For this review, take the finished solid that the model builds, in its own axes (mm). Round coordinates to 2 decimals unless told otherwise and drop trailing zeros. Order: outer loops, then holes, each group sorted by start corner. A loop starts at its lowest first (then second) coordinate and runs counter-clockwise, first axis right, second up. Notation, with made-up numbers: (79.25, 76.25) -> (133.25, 76.25) arc R32 ccw to (133.25, 113.25) -> close; hole circle Ø3 at (46, 35). An arc over 180 degrees is marked (long way). Use a Markdown table: item, result. Add a question column.
1) Consider section C-C (x = -23). State the section outline as (y, z) points.
2) Wall thickness on line 1 along Y through (x, z) = (-12.5, 5); line 2 along X through (y, z) = (-17, 3.45); line 3 along Y through (x, z) = (-3, 2.75): over which ranges is each line inside the solid? List them lowest first. Write a range as [from, to].
3) Consider section B-B (y = -16). State the section outline as (x, z) points, plus the area to 3 significant figures.
4) Consider section A-A (z = 3.65). State the section outline as (x, y) points, plus the area to 3 significant figures.
5) Clearance check with flat-ended pins moving along their axes: P1, Ø2, axis at y = 22, z = 2, coming from the +X side; P2, Ø12, axis at x = 21.65, y = -12.5, coming from the +Z side. State where each tip first meets the part, or that it passes through.
6) Draft analysis for pull direction X (two halves, no side actions). For faces 1 (the face through (-29.55, -18.55, 2.96)), 2 (the face through (3, 11, 6)), 3 (the face through (13.75, -18.55, 2.96)), state which applies: pulls with the +X half, pulls with the -X half, needs draft (parallel to the pull), parting line crosses it, or undercut.
7) Consider section D-D (y = 7). State the section outline as (x, z) points, plus the area to 3 significant figures.
```python
from build123d import *

# Parameters (mm, degrees)
F0_R     = 9.95
F1_DEPTH = 6


with BuildPart() as f1:
    # F0 (on Top) → F1 (new body)
    with BuildSketch(Plane.XY):
        with BuildLine():
            ThreePointArc((0, 11), (-7.778175, -7.778175), (11, 0))
            ThreePointArc((11, 0), (7.778175, 7.778175), (0, 11))
        make_face()
        with BuildLine():
            ThreePointArc((9.95, 25), (-7.035712, 32.035712), (0, 15.05))
            ThreePointArc((0, 15.05), (7.035712, 17.964288), (9.95, 25))
        make_face()
        with BuildLine():
            ThreePointArc((8.291562, 12.5), (0, 40), (-8.291562, 12.5))
            ThreePointArc((-8.291562, 12.5), (-12.990381, 7.5), (-14.971099, 0.930703))
            ThreePointArc((-14.971099, 0.930703), (-34.641016, -20), (-6.679537, -13.430703))
            ThreePointArc((-6.679537, -13.430703), (0, -15), (6.679537, -13.430703))
            ThreePointArc((6.679537, -13.430703), (34.641016, -20), (14.971099, 0.930703))
            ThreePointArc((14.971099, 0.930703), (12.990381, 7.5), (8.291562, 12.5))
        make_face()
        with Locations((-21.650635, -12.5)):
            Circle(F0_R, mode=Mode.SUBTRACT)
        with Locations((21.650635, -12.5)):
            Circle(F0_R, mode=Mode.SUBTRACT)
        with BuildLine():
            ThreePointArc((0, 11), (7.778175, 7.778175), (11, 0))
            ThreePointArc((11, 0), (-7.778175, -7.778175), (0, 11))
        make_face(mode=Mode.SUBTRACT)
        with BuildLine():
            ThreePointArc((9.95, 25), (7.035712, 17.964288), (0, 15.05))
            ThreePointArc((0, 15.05), (-7.035712, 32.035712), (9.95, 25))
        make_face(mode=Mode.SUBTRACT)
    extrude(amount=F1_DEPTH)


solid = f1.part
```
Results list:
| question | item | result |
|---|---|---|
| 1 | outline | (-27.44, 0) -> (-22.36, 0) -> (-22.36, 6) -> (-27.44, 6) -> close; (-2.64, 0) -> (2.44, 0) -> (2.44, 6) -> (-2.64, 6) -> close |
| 2 | line 1 | [-24.39, -16.41], [-8.59, 8.29], [16.71, 33.29] |
| 2 | line 2 | [-35.96, -30.52], [-12.78, -7.34], [7.34, 12.78], [30.52, 35.96] |
| 2 | line 3 | [-14.7, -10.58], [10.58, 15.51], [34.49, 39.7] |
| 3 | outline | (-36.24, 0) -> (-30.96, 0) -> (-30.96, 6) -> (-36.24, 6) -> close; (-12.34, 0) -> (-7.06, 0) -> (-7.06, 6) -> (-12.34, 6) -> close; (7.06, 0) -> (12.34, 0) -> (12.34, 6) -> (7.06, 6) -> close; (30.96, 0) -> (36.24, 0) -> (36.24, 6) -> (30.96, 6) -> close |
| 3 | area | 127 mm2 |
| 4 | outline | (-14.97, 0.93) arc R15 ccw (long way) to (-6.68, -13.43) arc R15 ccw to (6.68, -13.43) arc R15 ccw (long way) to (14.97, 0.93) arc R15 ccw to (8.29, 12.5) arc R15 ccw (long way) to (-8.29, 12.5) arc R15 ccw to start; hole circle Ø19.9 at (-21.65, -12.5); hole (0, 11) arc R11 ccw (long way) to (11, 0) arc R11 ccw to start; hole (0, 15.05) arc R9.95 ccw to (9.95, 25) arc R9.95 ccw (long way) to start; hole circle Ø19.9 at (21.65, -12.5) |
| 4 | area | 1,350 mm2 |
| 5 | P1 | x = 14.87 |
| 5 | P2 | through |
| 6 | face 1 | undercut |
| 6 | face 2 | needs draft |
| 6 | face 3 | undercut |
| 7 | outline | (-13.27, 0) -> (-8.49, 0) -> (-8.49, 6) -> (-13.27, 6) -> close; (8.49, 0) -> (13.27, 0) -> (13.27, 6) -> (8.49, 6) -> close |
| 7 | area | 57.4 mm2 |
